Verification items for the finished model (mm, model axes). A direction names the side the tool comes from. Coordinates: 2 decimals unless noted, no trailing zeros. Write each loop counter-clockwise with the first axis right and the second up, starting at its lowest first coordinate (ties: lowest second). Pieces come first, ordered by that corner, then holes. Notation, with made-up numbers: (-26, -25) - (23, -25) arc R25 ccw to (23, -8) - close; hole circle Ø2 at (83, 54.5). An arc over 180 degrees is marked (long way). Use one line per item in the form item = value. Start each with the question number.
(1) Gauge pin test, flat ends, axial feed: pin 1 Ø1.5 at (y, z) = (10, 31.5) entering from -X; pin 2 Ø1 at (x, y) = (5, 11.5) entering from +Z; pin 3 Ø10 at (y, z) = (33.5, 35) entering from -X. Record the tip position at first contact, or that the pin passes through.
(2) Mould release check, pull along X, two halves, no side actions. Record for faces 3 (the flat face through (-33, 50.8, 20)), 4 (the cylindrical face through (38.93, 1.61, 44.87)), 5 (the cylindrical face through (-35.19, 1.61, 44.6)), 6 (the cylindrical face through (5.79, 25.04, -44.07)): released by +X, released by -X, zero draft, split by the parting line, or undercut.
(3) Sectioned sample at C-C (y = 46). Record the cut outline in (x, z), and give its area (3 significant figures).
(4) Tool access check on faces 1 (the flat face through (1, 3.175, 48)), 2 (the flat face through (-44.45, 2, 28)). Record the directions out of +Z, -Z, +X, -X, +Y, -Y that give a thin tool (end or side, any length) a straight path to the whole face; none if there is none.
(5) Material ranges on line 1 (Z direction, x = 0, y = 1.55); line 2 (X direction, y = 34.5, z = -8); line 3 (Y direction, x = 7, z = 44) (3 decimals), recorded low to high. Write a range as [from, to].
(6) Sectioned sample at A-A (x = 0). Record the cut outline in (y, z) (3 decimals), and give its area (3 significant figures).
(7) Sectioned sample at D-D (z = -30). Record the cut outline in (x, y), and give its area (3 significant figures).
(8) Sectioned sample at B-B (z = -15). Record the cut outline in (x, y), and give its area (3 significant figures).
Autodesk Inventor part; units mm, degrees
ref_plane "YZ Plane" through (0, 0, 0) normal (1, 0, 0) x (0, 1, 0)
ref_plane "XZ Plane" through (0, 0, 0) normal (0, 1, 0) x (-1, 0, 0)
ref_plane "XY Plane" through (0, 0, 0) normal (0, 0, 1) x (1, 0, 0)
sketch "Sketch1" plane through (0, 0, 0) normal (0, 1, 0) x (-1, 0, 0)
  circle A0 centre (0, 0) radius 38.1
  circle A1 centre (0, 0) radius 44.45
  dimension "d0" = 76.2
  dimension "d1" = 88.9
sketch "Sketch2" plane through (0, 0, 0) normal (0, 1, 0) x (-1, 0, 0)
  circle A0 centre (0, 0) radius 44.45
  line L0 (44.45, 0) -> (44.45, 57.15)
  line L1 (-44.45, 0) -> (-44.45, 57.15)
  line L2 (-44.45, 57.15) -> (44.45, 57.15)
  dimension "d8" = 57.15
extrude "Extrusion1" add sketch "Sketch1" along normal blind 50.8
extrude "Extrusion2" add sketch "Sketch2" along normal blind 3.175
sketch "Sketch3" plane through (0, 3.175, 0) normal (0, 1, 0) x (1, 0, 0)
  circle A0 centre (0, 0) radius 38.1
extrude "Extrusion3" cut sketch "Sketch3" against normal blind 3.175
sketch "Sketch4" plane through (0, 3.175, 0) normal (0, 1, 0) x (1, 0, 0)
  circle A0 centre (-36.068, -45.974) radius 1.6319
  line L0 (-44.45, 0) -> (-44.45, -57.15)
  line L1 (-44.45, -57.15) -> (44.45, -57.15)
  circle A1 centre (40.132, -45.974) radius 1.6319
  point P0 (0, 0)
  dimension "d11" = 3.2639
  dimension "d12" = 8.382
  dimension "d13" = 11.176
  dimension "d14" = 3.2639
  dimension "d15" = 76.2
  dimension "d16" = 0
extrude "Extrusion4" cut sketch "Sketch4" against normal blind 3.175
properties part number "Battery_holder2"
Answers below:
q1.pin_1 = -32.1
q1.pin_2 = 44.22
q1.pin_3 = -32.8
q2.face_3 = zero draft
q2.face_4 = undercut
q2.face_5 = undercut
q2.face_6 = split by the parting line
q3.outline = circle Ø88.9 at (0, 0); hole circle Ø76.2 at (0, 0)
q3.area = 1,650 mm2
q4.face_1 = +Z, +Y
q4.face_2 = +Z, -Z, -X, +Y, -Y
q5.line_1 = [-44.45, -38.1], [38.1, 57.15]
q5.line_2 = [-43.72, -37.25], [37.25, 43.72]
q5.line_3 = [0, 3.175]
q6.outline = (0, -44.45) - (50.8, -44.45) - (50.8, -38.1) - (0, -38.1) - close; (0, 38.1) - (50.8, 38.1) - (50.8, 44.45) - (3.175, 44.45) - (3.175, 57.15) - (0, 57.15) - close
q6.area = 685 mm2
q7.outline = (-32.8, 0) - (-23.49, 0) - (-23.49, 50.8) - (-32.8, 50.8) - close; (23.49, 0) - (32.8, 0) - (32.8, 50.8) - (23.49, 50.8) - close
q7.area = 946 mm2
q8.outline = (-41.84, 0) - (-35.02, 0) - (-35.02, 50.8) - (-41.84, 50.8) - close; (35.02, 0) - (41.84, 0) - (41.84, 50.8) - (35.02, 50.8) - close
q8.area = 693 mm2
